```python
from build123d import *

# Parameters (mm, degrees)
F0_W     = 9.11
F0_H     = 11.21
F1_DEPTH = 0.6
F2_DEPTH = 1.2


with BuildPart() as f1:
    # F0 (on Top) → F1 (new body)
    with BuildSketch(Plane.XY):
        Polygon((11.11, 0), (0, 0), (0, -12.21), (1, -12.21), (1, -1), (10.11, -1), (10.11, -12.21), (11.11, -12.21), align=None)
        with Locations((5.555, -6.605)):
            Rectangle(F0_W, F0_H)
    extrude(amount=-F1_DEPTH)

    # F0 (on Top) → F2 (join)
    with BuildSketch(Plane.XY):
        Polygon((11.11, 0), (0, 0), (0, -12.21), (1, -12.21), (1, -1), (10.11, -1), (10.11, -12.21), (11.11, -12.21), align=None)
    extrude(amount=F2_DEPTH)


solid = f1.part
```
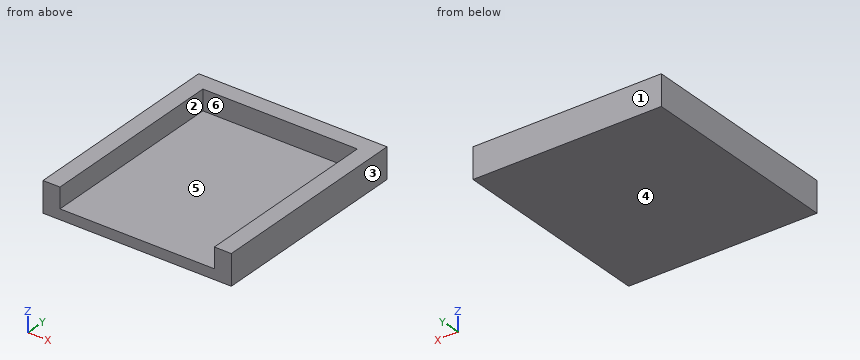
Part model, mm, in its own coordinate system. Face numbers are marked on the shaded views. A direction names the side the tool comes from. Give positions to 0.01 mm unless a question says otherwise; leave off trailing zeros. Order: outer loops, then holes, each group sorted by start corner. A loop starts at its lowest first (then second) coordinate and runs counter-clockwise, first axis right, second up. Notation, with made-up numbers: M -28.5,-21.75 L -23.5,-21.75 A14 ccw -23.5,-14.75 Z; hole C 37,-17 d6. An arc over 180 degrees is marked long. Use a Markdown table: item, result. Add a question column.
(1) Drop flat-ended pins along their axis: P1, Ø0.6, axis at y = -8, z = 1, coming from the -X side; P2, Ø1, axis at x = 6, z = 1, coming from the -Y side. Give the stop position or say it passes through.
(2) Saw through at B-B, the plane z = 0.6. Give the cut face in (x, y).
(3) Mould opens along X. For the marked faces 3, 4, 5 and 6 say: +X half, -X half, draft (parallel to the pull), parting line (faces both ways), or undercut.
(4) Saw through at A-A, the plane y = -3.5. Give the cut face in (x, z).
(5) 3-axis set-ups, long thin cutter, end or side, ignore diameter. For the marked faces 1 and 2: which of +Z, -Z, +X, -X, +Y, -Y reach the whole face in a straight line?
(6) Saw through at C-C, the plane x = 8. Give the cut face in (y, z), and give its area (3 significant figures).
(7) Probe line 1 along X through (y, z) = (-10, 0.2); line 2 along Y through (x, z) = (4.25, 0.1); line 3 along Z through (x, y) = (9, -8.5). List the from-to ranges inside material, lowest first. Write a range as [from, to].
Answer key:
| question | item | result |
|---|---|---|
| 1 | P1 | x = 0 |
| 1 | P2 | y = -1 |
| 2 | outline | M 0,-12.21 L 1,-12.21 L 1,-1 L 10.11,-1 L 10.11,-12.21 L 11.11,-12.21 L 11.11,0 L 0,0 Z |
| 3 | face 3 | +X half |
| 3 | face 4 | draft |
| 3 | face 5 | undercut |
| 3 | face 6 | undercut |
| 4 | outline | M 0,-0.6 L 11.11,-0.6 L 11.11,1.2 L 10.11,1.2 L 10.11,0 L 1,0 L 1,1.2 L 0,1.2 Z |
| 5 | face 1 | +Z, -Z, +X, -X, +Y |
| 5 | face 2 | +Z, -Y |
| 6 | outline | M -12.21,-0.6 L 0,-0.6 L 0,1.2 L -1,1.2 L -1,0 L -12.21,0 Z |
| 6 | area | 8.53 mm^2 |
| 7 | line 1 | [0, 1], [10.11, 11.11] |
| 7 | line 2 | [-1, 0] |
| 7 | line 3 | [-0.6, 0] |
